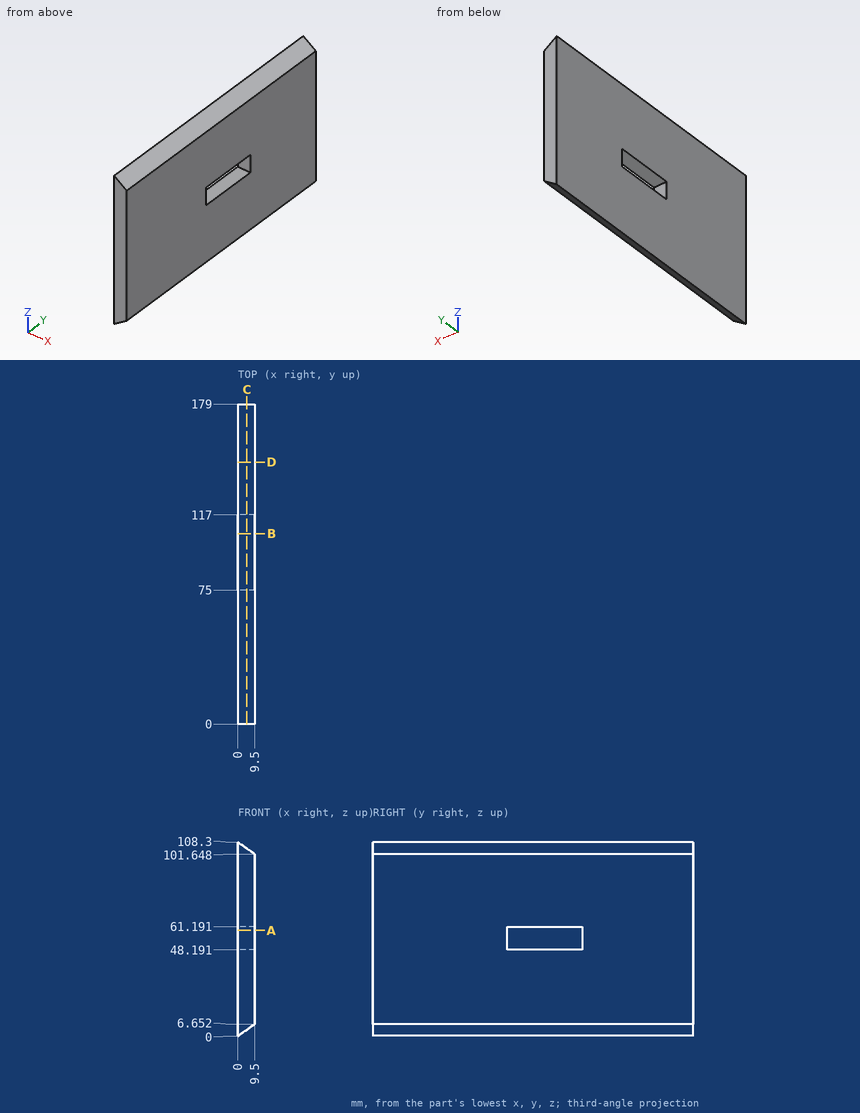
Answer from the drawing. Dimensions are ordinates in mm from the lowest x, y and z of the part. Give positions to 0.01 mm unless a question says otherwise; leave off trailing zeros. Write each loop counter-clockwise with the first axis right and the second up, starting at its lowest first coordinate (ties: lowest second). Pieces come first, ordered by that corner, then holes. Notation, with made-up numbers: (54.25, 11) -> (95.25, 11) arc R37 cw to (95.25, 50) -> close; hole circle Ø11 at (12.5, 36). An arc over 180 degrees is marked (long way). One line per question, with ' | ' between items. Start each with the question number.
1. Given pin 1 Ø2 at (x, y) = (2.5, 134) entering from -Z; pin 2 Ø4 at (x, y) = (5.5, 24) entering from +Z; pin 3 Ø5 at (x, y) = (5.5, 89) entering from +Z, each flat-ended and moving along its own axis, determine where each tip first touches the part or whether it passes through.
2. Section D-D (y = 146.5) is taken. Determine the outline of the cut face in (x, z).
3. Section B-B (y = 106.5) is taken. Determine the outline of the cut face in (x, z).
4. Section C-C (x = 5) is taken. Determine the outline of the cut face in (y, z), plus the area to 3 significant figures.
5. Section A-A (z = 59) is taken. Determine the outline of the cut face in (x, y).
6. Find the intervals of material crossed by probe 1 along Z at (x, y) = (4.5, 97.5); probe 2 along Z at (x, y) = (8.5, 11.5); probe 3 along Z at (x, y) = (8.5, 92.5), in increasing order.
Response values:
1) pin 1: z = 1.05 | pin 2: z = 105.85 | pin 3: z = 106.2
2) outline: (0, 0) -> (9.5, 6.65) -> (9.5, 101.65) -> (0, 108.3) -> close
3) outline: (0, 0) -> (9.5, 6.65) -> (9.5, 48.19) -> (0, 48.19) -> close; (0, 61.19) -> (9.5, 61.19) -> (9.5, 101.65) -> (0, 108.3) -> close
4) outline: (0, 3.5) -> (179, 3.5) -> (179, 104.8) -> (0, 104.8) -> close; hole (75, 48.19) -> (117, 48.19) -> (117, 61.19) -> (75, 61.19) -> close | area: 17,600 mm2
5) outline: (0, 0) -> (9.5, 0) -> (9.5, 75) -> (0, 75) -> close; (0, 117) -> (9.5, 117) -> (9.5, 179) -> (0, 179) -> close
6) probe 1: 3.15 to 48.19, 61.19 to 105.15 | probe 2: 5.95 to 102.35 | probe 3: 5.95 to 48.19, 61.19 to 102.35
